Autodesk Inventor part; units mm, degrees
ref_plane "YZ Plane" through (0, 0, 0) normal (1, 0, 0) x (0, 1, 0)
ref_plane "XZ Plane" through (0, 0, 0) normal (0, 1, 0) x (-1, 0, 0)
ref_plane "XY Plane" through (0, 0, 0) normal (0, 0, 1) x (1, 0, 0)
sketch "스케치1" plane through (0, 0, 0) normal (0, 1, 0) x (-1, 0, 0)
  line L0 (14.7, -17.45) -> (14.7, -23.65)
  line L1 (-14.7, -23.65) -> (-14.7, -17.45)
  line L2 (-14.7, -17.45) -> (-20.25, -17.45)
  line L3 (-20.25, -17.45) -> (-20.25, 16.75)
  line L4 (-20.25, 16.75) -> (-14.7, 16.75)
  line L5 (-14.7, 16.75) -> (-14.7, 22.95)
  line L6 (14.7, 22.95) -> (14.7, 16.75)
  line L7 (14.7, 16.75) -> (20.45, 16.75)
  line L8 (20.45, 16.75) -> (20.45, -17.45)
  line L9 (20.45, -17.45) -> (14.7, -17.45)
  line L10 (-14.7, -23.65) -> (-18.4575, -23.65)
  line L11 (14.7, -23.65) -> (18.4575, -23.65)
  line L12 (14.7, 22.95) -> (19.3209, 22.95)
  line L13 (-14.7, 22.95) -> (-19.3209, 22.95)
  arc A0 (-19.3209, 22.95) -> (-18.4575, -23.65) centre (0, 0) ccw
  arc A1 (18.4575, -23.65) -> (19.3209, 22.95) centre (0, 0) ccw
  line L14 (-18.4575, -23.65) -> (-14.7, -23.65)
  line L15 (14.7, -23.65) -> (18.4575, -23.65)
  point P0 (-20, 0)
  point P1 (-30, 0)
  dimension "d12" = 40.7
  dimension "d13" = 34.2
extrude "돌출1" add sketch "스케치1" along normal blind 5
sketch "스케치2" plane through (0, 5, 0) normal (0, 1, 0) x (1, 0, 0)
  line L0 (-14.7, 23.65) -> (-18.4575, 23.65)
  arc A0 (-18.4575, 23.65) -> (-19.3209, -22.95) centre (0, 0) ccw
  line L1 (-19.3209, -22.95) -> (-14.7, -22.95)
  line L2 (-14.7, -22.95) -> (-14.7, -16.75)
  line L3 (-14.7, -16.75) -> (-20.45, -16.75)
  line L4 (-20.45, -16.75) -> (-20.45, 17.45)
  line L5 (-20.45, 17.45) -> (-14.7, 17.45)
  line L6 (-14.7, 17.45) -> (-14.7, 23.65)
  line L7 (18.4575, 23.65) -> (14.7, 23.65)
  line L8 (14.7, 23.65) -> (14.7, 17.45)
  line L9 (14.7, 17.45) -> (20.25, 17.45)
  line L10 (20.25, 17.45) -> (20.25, -16.75)
  line L11 (20.25, -16.75) -> (14.7, -16.75)
  line L12 (14.7, -16.75) -> (14.7, -22.95)
  line L13 (14.7, -22.95) -> (19.3209, -22.95)
  arc A1 (19.3209, -22.95) -> (18.4575, 23.65) centre (0, 0) ccw
  line L14 (14.7, -22.95) -> (-14.7, -22.95)
  line L15 (-14.7, 23.65) -> (14.7, 23.65)
extrude "돌출2" add sketch "스케치2" along normal blind 10
fillet "모깎기1" radius 15 4 edges at (-29.9949, 15, -0.5558) (29.9949, 15, -0.5558) (0, 15, 22.95) (0, 15, -23.65)
sketch "스케치3" plane through (0, 5, 0) normal (0, -1, 0) x (1, 0, 0)
  line L0 (-14.7, 22.0921) -> (14.7, 22.0921)
  line L1 (-14.7, 22.0921) -> (-14.7, 16.75)
  line L2 (-14.7, 16.75) -> (-20.45, 16.75)
  line L3 (-20.45, 16.75) -> (-20.45, -17.45)
  line L4 (-20.45, -17.45) -> (-14.7, -17.45)
  line L5 (-14.7, -17.45) -> (-14.7, -22.7921)
  line L6 (14.7, -22.7921) -> (-14.7, -22.7921)
  line L7 (14.7, -22.7921) -> (14.7, -17.45)
  line L8 (14.7, -17.45) -> (20.25, -17.45)
  line L9 (20.25, -17.45) -> (20.25, 16.75)
  line L10 (20.25, 16.75) -> (14.7, 16.75)
  line L11 (14.7, 16.75) -> (14.7, 22.0921)
  line L12 (20.25, 16.75) -> (-20.45, 16.75)
  line L13 (-20.45, 16.75) -> (-20.45, 12.75)
  line L14 (-20.45, 12.75) -> (20.25, 12.75)
  line L15 (20.25, 12.75) -> (20.25, 16.75)
  line L16 (20.25, -17.45) -> (-20.45, -17.45)
  line L17 (-20.45, -17.45) -> (-20.45, -12.75)
  line L18 (-20.45, -12.75) -> (20.25, -12.75)
  line L19 (20.25, -12.75) -> (20.25, -17.45)
  line L20 (20.25, 12.75) -> (16.25, 12.75)
  line L21 (16.25, 12.75) -> (16.25, -12.75)
  line L22 (16.25, -12.75) -> (20.25, -12.75)
  line L23 (20.25, -12.75) -> (20.25, 12.75)
  line L24 (-20.45, 12.75) -> (-16.45, 12.75)
  line L25 (-16.45, 12.75) -> (-16.45, -12.75)
  line L26 (-16.45, -12.75) -> (-20.45, -12.75)
  line L27 (-20.45, -12.75) -> (-20.45, 12.75)
  point P0 (0, 0)
  point P1 (-16.45, 12.75)
  point P2 (20.25, -12.75)
  point P3 (20.25, 12.75)
  dimension "d5" = 4
  dimension "d6" = 4.7
  dimension "d7" = 4
  dimension "d8" = 4
extrude "돌출3" add sketch "스케치3" along normal blind 20 contours L14 L25 L18 L3 | L9 L18 L21 L14
fillet "모깎기2" radius 2 8 edges at (16.25, -15, 0) (18.25, -15, 12.75) (20.25, -15, 0) (18.25, -15, -12.75) (-16.45, -15, 0) (-18.45, -15, 12.75) (-20.45, -15, 0) (-18.45, -15, -12.75)
sketch "스케치4" plane through (16.25, 5, -12.75) normal (-1, 0, 0) x (0, 0, 1)
  line L0 (0, -18) -> (25.5, -18)
  line L1 (0, -5) -> (0, -18)
  line L2 (0, -5) -> (25.5, -5)
  line L3 (25.5, -5) -> (25.5, -18)
  line L4 (29.5, -5) -> (29.5, 0)
  line L5 (29.5, 0) -> (15.5, 0)
  line L6 (15.5, 0) -> (15.5, -23.2577)
  line L7 (15.5, -23.2577) -> (29.5, -23.2577)
  line L8 (29.5, -23.2577) -> (29.5, 0)
  point P0 (12.75, -5)
  dimension "d14" = 14
extrude "돌출4" cut sketch "스케치4" against normal blind 20 contours L6 L2 L3 L0 | L0 L3 L2 L6 L5 L4 L8 L7
properties part number "arm cover1"
Work out the finished part from the listing and answer in its coordinate system (mm). A direction names the side the tool comes from. Give positions to 0.01 mm unless a question says otherwise; leave off trailing zeros. Write each loop counter-clockwise with the first axis right and the second up, starting at its lowest first coordinate (ties: lowest second). Pieces come first, ordered by that corner, then holes.
Q1. The part is cut by section A-A on y = -8. Give the vertices of the cut face in (x, z), and give its area (3 significant figures).
Answer:
outline: (-20.45, -12.75) - (-16.45, -12.75) - (-16.45, 12.75) - (-20.45, 12.75) - close; (16.25, -12.75) - (20.25, -12.75) - (20.25, 2.75) - (16.25, 2.75) - close
area: 164 mm2
Q2. Straight lines are drawn through the part: L1, parallel to X at y = -8, z = -9; L2, parallel to Z at x = -18.5, y = -3.5; L3, parallel to Y at x = -6, z = -5. For each, find the intervals that lie inside material, in ascending order.
Answer:
L1: x = -20.45 to -16.45, 16.25 to 20.25
L2: z = -12.75 to 12.75
L3: y = 5 to 15
Q3. The part is cut by section C-C on y = 2.5. State how many separate pieces and enclosed holes the cut face has, and give its area (3 significant figures).
Answer:
separate pieces: 3
enclosed holes: 0
area: 757 mm2
Q4. Given pin 1 (4.5 mm diameter, centred on x = 17.5, y = -4.5, fed in from -Z); pin 2 (22.5 mm diameter, centred on x = -0.5, z = 3.5, fed in from -Y); pin 3 (9 mm diameter, centred on y = -1, z = -2, fed in from +X); pin 4 (7 mm diameter, centred on x = 20, z = 18.5, fed in from -Y), each flat-ended and moving along its own axis, determine where each tip first touches the part or whether it passes through.
Answer:
pin 1: stops at z = -12.75
pin 2: stops at y = 5
pin 3: stops at x = 30
pin 4: stops at y = 0
Q5. A tool of negligible diameter and unlimited length cuts with its end or side. For faces 5 (the face through (14.7, 2, -21)), 6 (the face through (19, 0, 19)), 7 (the face through (20.25, 2, -15)), 8 (the face through (-20.45, 2, 15)), from which of +Z, -Z, +X, -X, +Y, -Y can it reach the whole face along a straight path? Write none if from no direction.
Answer:
face 5: +Z, -Z, -Y
face 6: +Z, +X, -X, -Y
face 7: -Y
face 8: +X, -Y
Q6. The part is cut by section B-B on x = -9.5. Give the vertices of the cut face in (y, z), and give its area (3 significant figures).
Answer:
outline: (5, -22.79) arc R15 ccw to (15, -8.65) - (15, 7.95) arc R15 ccw to (5, 22.09) - close
area: 372 mm2
Q7. For a pull along Z with two mould halves and no side action, classify faces 1 (the face through (18, -4, -12.75)), 2 (the face through (-20.45, -6, 0)), 3 (the face through (0.27, 10.72, 18.44)), 4 (the face through (4, 5, -1)) as released by +Z, released by -Z, zero draft, split by the parting line, or undercut.
Answer:
face 1: undercut
face 2: zero draft
face 3: released by +Z
face 4: undercut
